from build123d import *

# Parameters (mm, degrees)
BOSS_EXTRUDE1_DEPTH = 50.8
SKETCH4_R           = 1.4732
CUT_EXTRUDE1_DEPTH  = 11.16
SKETCH5_R           = 3.2131
SKETCH5_R_2         = 5.1308
CUT_EXTRUDE2_DEPTH  = 50.8


with BuildPart() as part:
    # Sketch3 → Boss-Extrude1 (new body)
    with BuildSketch(Plane(origin=(0, 0, 0), x_dir=(0, 0, -1), z_dir=(1, 0, 0))):
        Polygon((0, 0), (25.4, 0), (25.4, 25.4), (13.97, 25.4), (13.97, 10.16), (0, 10.16), align=None)
    extrude(amount=-BOSS_EXTRUDE1_DEPTH)

    # Sketch4 → Cut-Extrude1 (cut, through all)
    with BuildSketch(Plane(origin=(0, 10.16, 0), x_dir=(1, 0, 0), z_dir=(0, 1, 0))):
        with Locations((-44.45, 6.35)):
            Circle(SKETCH4_R)
        with Locations((-22.098, 6.35)):
            Circle(SKETCH4_R)
    extrude(amount=-CUT_EXTRUDE1_DEPTH, mode=Mode.SUBTRACT)

    # Sketch5 → Cut-Extrude2 (cut)
    with BuildSketch(Plane.XY.offset(-13.97)):
        with Locations((-38.1, 19.05)):
            Circle(SKETCH5_R)
        with Locations((-12.7, 19.05)):
            Circle(SKETCH5_R_2)
    extrude(amount=-CUT_EXTRUDE2_DEPTH, mode=Mode.SUBTRACT)


solid = part.part
Geometry: final body of the model. Coordinates: model frame, mm. A direction names the side the tool comes from. Round coordinates to 2 decimals unless told otherwise and drop trailing zeros. Loops run counter-clockwise (first coordinate to the right, second up) from the corner with the lowest first, then second, coordinate; pieces in that order, holes last. Notation, with made-up numbers: M 89.25,19 L 105.25,19 A9 cw 105.25,24 Z; hole C 21.25,1 d5. An arc over 180 degrees is marked long. Put each result on its own line as item: value. Start each with the question number.
(1) Draft query along X for faces 3 (the face through (-25, 25.4, -20)), 4 (the face through (-35.13, 17.82, -19.6)), 5 (the face through (-23.18, 5.15, -7.35)), 6 (the face through (-50.8, 10, -15)). Return one class per face: +X half, -X half, draft (parallel to the pull), parting line (faces both ways), or undercut.
(2) Contact query for flat-ended pins moving along their axis: pin 1 Ø1 at (x, z) = (-43, -8.5) entering from +Y; pin 2 Ø2 at (x, y) = (-44, 20.5) entering from +Z. Output: stop coordinate, or through.
(3) Section query B-B (z = -6.35). Return loops of the section in (x, y).
(4) Section query A-A (x = -38.1). Return loops of the section in (y, z), then the cut area to 3 significant figures.
(5) Set-up query: faces 1 (the face through (-25, 18, -13.97)), 2 (the face through (-25, 0, -13)). Return all of +Z, -Z, +X, -X, +Y, -Y with unobstructed straight access to the full face (end or side cutting, diameter ignored); none if empty.
(6) Section query D-D (x = -44.45). Return loops of the section in (y, z), then the cut area to 3 significant figures.
(7) Material intervals for line 1 along X through (y, z) = (3, -6.35); line 2 along X through (y, z) = (6.25, -6); line 3 along Z through (x, y) = (-44.45, 7), sorted ascending. Write a range as [from, to].
(8) Section query C-C (y = 19.05). Return loops of the section in (x, z), then the cut area to 3 significant figures.
Findings below:
1. face 3: draft
1. face 4: undercut
1. face 5: undercut
1. face 6: -X half
2. pin 1: stops at y = 10.16
2. pin 2: stops at z = -13.97
3. outline: M -50.8,0 L -45.92,0 L -45.92,10.16 L -50.8,10.16 Z; M -42.98,0 L -23.57,0 L -23.57,10.16 L -42.98,10.16 Z; M -20.62,0 L 0,0 L 0,10.16 L -20.62,10.16 Z
4. outline: M 0,-25.4 L 15.84,-25.4 L 15.84,-13.97 L 10.16,-13.97 L 10.16,0 L 0,0 Z; M 22.26,-25.4 L 25.4,-25.4 L 25.4,-13.97 L 22.26,-13.97 Z
4. area: 359 mm2
5. face 1: +Z, +X, -X, +Y
5. face 2: +Z, -Z, +X, -X, -Y
6. outline: M 0,-25.4 L 25.4,-25.4 L 25.4,-13.97 L 10.16,-13.97 L 10.16,-7.82 L 0,-7.82 Z; M 0,-4.88 L 10.16,-4.88 L 10.16,0 L 0,0 Z
6. area: 402 mm2
7. line 1: x = [-50.8, -45.92], [-42.98, -23.57], [-20.62, 0]
7. line 2: x = [-50.8, -45.88], [-43.02, -23.53], [-20.67, 0]
7. line 3: z = [-25.4, -7.82], [-4.88, 0]
8. outline: M -50.8,-25.4 L -41.31,-25.4 L -41.31,-13.97 L -50.8,-13.97 Z; M -34.89,-25.4 L -17.83,-25.4 L -17.83,-13.97 L -34.89,-13.97 Z; M -7.57,-25.4 L 0,-25.4 L 0,-13.97 L -7.57,-13.97 Z
8. area: 390 mm2
